For this review, take the finished solid that the model builds, in its own axes (mm). Coordinates: 2 decimals unless noted, no trailing zeros. Loops run counter-clockwise (first coordinate to the right, second up) from the corner with the lowest first, then second, coordinate; pieces in that order, holes last. Notation, with made-up numbers: (-6, 49) - (22, 49) arc R13 ccw to (22, 63) - close; hole circle Ø9 at (86.25, 42). An arc over 180 degrees is marked (long way). One line per item, written item: value. Start each with the question number.
1. Insertion check: pin 1 (1.1 mm diameter, centred on y = -11, z = 2, fed in from -X); pin 2 (4.5 mm diameter, centred on x = -129.33, y = 110, fed in from -Z); pin 3 (2 mm diameter, centred on y = 57, z = 1.5, fed in from +X). Each pin has a flat end and moves straight along its axis. Give the tip position at first contact, or say it passes through.
2. Take a section at D-D, the plane y = -95. State the section outline as (x, z) points, and give its area (3 significant figures).
3. Take a section at C-C, the plane z = 2.8. Count the separate pieces of the cut face and the enclosed holes in it, and give its area (3 significant figures).
4. Take a section at A-A, the plane y = 0. State the section outline as (x, z) points.
5. Take a section at B-B, the plane x = -3. State the section outline as (y, z) points.
6. To check wall thickness, follow line 1 (X direction, y = -18.5, z = 2.4); line 2 (Y direction, x = -54.06, z = 2.8) (3 decimals); line 3 (X direction, y = 25.5, z = 2.3). State the ranges of each line that lie inside material, in increasing order. Write a range as from..to.
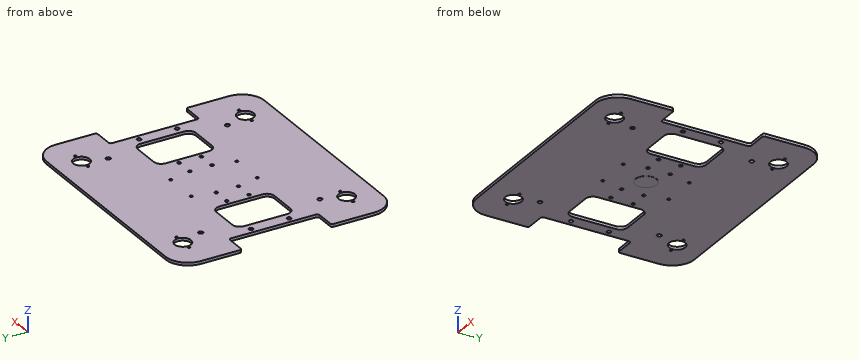
```python
from build123d import *

# Parameters (mm, degrees)
SKETCH2_R                      = 1.65
SKETCH2_R_2                    = 11
SKETCH2_R_3                    = 3
SKETCH2_R_4                    = 1.9
SKETCH2_R_5                    = 2.25
BOSS_EXTRUDE1_DEPTH            = 3.8
M5_CLEARANCE_HOLE1_D           = 5.5
M5_CLEARANCE_HOLE1_CSINK_D     = 5.55
M5_CLEARANCE_HOLE1_CSINK_ANGLE = 90
SKETCH4_R                      = 13.987722527
BOSS_EXTRUDE2_DEPTH            = 0.2


with BuildPart() as part:
    # Sketch2 → Boss-Extrude1 (new body)
    with BuildSketch(Plane.XY):
        with BuildLine():
            Line((165, 63), (165, 115))
            ThreePointArc((165, 115), (156.213203436, 136.213203436), (135, 145))
            Line((135, 145), (71.563974327, 145))
            Line((71.563974327, 145), (-71.563974327, 145))
            Line((-71.563974327, 145), (-135, 145))
            ThreePointArc((-135, 145), (-156.213203436, 136.213203436), (-165, 115))
            Line((-165, 115), (-165, 63))
            ThreePointArc((-165, 63), (-164.121320344, 60.878679656), (-162, 60))
            Line((-162, 60), (-138, 60))
            ThreePointArc((-138, 60), (-135.878679656, 59.121320344), (-135, 57))
            Line((-135, 57), (-135, -57))
            ThreePointArc((-135, -57), (-135.878679656, -59.121320344), (-138, -60))
            Line((-138, -60), (-162, -60))
            ThreePointArc((-162, -60), (-164.121320344, -60.878679656), (-165, -63))
            Line((-165, -63), (-165, -117.5))
            ThreePointArc((-165, -117.5), (-156.213203436, -138.713203436), (-135, -147.5))
            Line((-135, -147.5), (135, -147.5))
            ThreePointArc((135, -147.5), (156.213203436, -138.713203436), (165, -117.5))
            Line((165, -117.5), (165, -63))
            ThreePointArc((165, -63), (164.121320344, -60.878679656), (162, -60))
            Line((162, -60), (138, -60))
            ThreePointArc((138, -60), (135.878679656, -59.121320344), (135, -57))
            Line((135, -57), (135, 57))
            ThreePointArc((135, 57), (135.878679656, 59.121320344), (138, 60))
            Line((138, 60), (162, 60))
            ThreePointArc((162, 60), (164.121320344, 60.878679656), (165, 63))
        make_face()
        with Locations(Location((-129.334802826, -110, 0), (0, 0, 180))):
            Circle(SKETCH2_R, mode=Mode.SUBTRACT)
        with Locations(Location((-115, -110, 0), (0, 0, 180))):
            Circle(SKETCH2_R_2, mode=Mode.SUBTRACT)
        with Locations(Location((-100.665197174, -110, 0), (0, 0, 180))):
            Circle(SKETCH2_R, mode=Mode.SUBTRACT)
        with Locations(Location((-105, -80, 0), (0, 0, 180))):
            Circle(SKETCH2_R_3, mode=Mode.SUBTRACT)
        with Locations(Location((-127.121259344, -25.5, 0), (0, 0, 180))):
            Circle(SKETCH2_R, mode=Mode.SUBTRACT)
        with Locations(Location((-23.312977745, -44.325601579, 0), (0, 0, 180))):
            Circle(SKETCH2_R_4, mode=Mode.SUBTRACT)
        with Locations(Location((-54.06, -14.995, 0), (0, 0, 180))):
            Circle(SKETCH2_R_5, mode=Mode.SUBTRACT)
        with Locations(Location((-30, -14.995, 0), (0, 0, 180))):
            Circle(SKETCH2_R_5, mode=Mode.SUBTRACT)
        with Locations(Location((100.665197174, -110, 0), (0, 0, 180))):
            Circle(SKETCH2_R, mode=Mode.SUBTRACT)
        with Locations(Location((115, -110, 0), (0, 0, 180))):
            Circle(SKETCH2_R_2, mode=Mode.SUBTRACT)
        with Locations(Location((105, -80, 0), (0, 0, 180))):
            Circle(SKETCH2_R_3, mode=Mode.SUBTRACT)
        with Locations(Location((129.334802826, -110, 0), (0, 0, 180))):
            Circle(SKETCH2_R, mode=Mode.SUBTRACT)
        with Locations(Location((23.312977745, -44.325601579, 0), (0, 0, 180))):
            Circle(SKETCH2_R_4, mode=Mode.SUBTRACT)
        with Locations(Location((30, -14.995, 0), (0, 0, 180))):
            Circle(SKETCH2_R_5, mode=Mode.SUBTRACT)
        with Locations(Location((54.06, -14.995, 0), (0, 0, 180))):
            Circle(SKETCH2_R_5, mode=Mode.SUBTRACT)
        with Locations(Location((127.121259344, -25.5, 0), (0, 0, 180))):
            Circle(SKETCH2_R, mode=Mode.SUBTRACT)
        with Locations(Location((-127.121259344, 25.5, 0), (0, 0, 180))):
            Circle(SKETCH2_R, mode=Mode.SUBTRACT)
        with BuildLine():
            ThreePointArc((-117.12, 28.95), (-114.191067812, 36.021067812), (-107.12, 38.95))
            Line((-107.12, 38.95), (-71.12, 38.95))
            ThreePointArc((-71.12, 38.95), (-64.048932188, 36.021067812), (-61.12, 28.95))
            Line((-61.12, 28.95), (-61.12, -29.05))
            ThreePointArc((-61.12, -29.05), (-64.048932188, -36.121067812), (-71.12, -39.05))
            Line((-71.12, -39.05), (-107.12, -39.05))
            ThreePointArc((-107.12, -39.05), (-114.191067812, -36.121067812), (-117.12, -29.05))
            Line((-117.12, -29.05), (-117.12, 28.95))
        make_face(mode=Mode.SUBTRACT)
        with Locations(Location((-54.06, 14.895, 0), (0, 0, 180))):
            Circle(SKETCH2_R_5, mode=Mode.SUBTRACT)
        with Locations(Location((-30, 14.895, 0), (0, 0, 180))):
            Circle(SKETCH2_R_5, mode=Mode.SUBTRACT)
        with Locations(Location((-23.312977745, 44.325601579, 0), (0, 0, 180))):
            Circle(SKETCH2_R_4, mode=Mode.SUBTRACT)
        with Locations(Location((-105, 80, 0), (0, 0, 180))):
            Circle(SKETCH2_R_3, mode=Mode.SUBTRACT)
        with Locations(Location((-129.334802826, 110, 0), (0, 0, 180))):
            Circle(SKETCH2_R, mode=Mode.SUBTRACT)
        with Locations(Location((-115, 110, 0), (0, 0, 180))):
            Circle(SKETCH2_R_2, mode=Mode.SUBTRACT)
        with Locations(Location((-100.665197174, 110, 0), (0, 0, 180))):
            Circle(SKETCH2_R, mode=Mode.SUBTRACT)
        with Locations(Location((30, 14.895, 0), (0, 0, 180))):
            Circle(SKETCH2_R_5, mode=Mode.SUBTRACT)
        with Locations(Location((54.06, 14.895, 0), (0, 0, 180))):
            Circle(SKETCH2_R_5, mode=Mode.SUBTRACT)
        with Locations(Location((23.312977745, 44.325601579, 0), (0, 0, 180))):
            Circle(SKETCH2_R_4, mode=Mode.SUBTRACT)
        with BuildLine():
            Line((61.12, -29.05), (61.12, 28.95))
            ThreePointArc((61.12, 28.95), (64.048932188, 36.021067812), (71.12, 38.95))
            Line((71.12, 38.95), (107.12, 38.95))
            ThreePointArc((107.12, 38.95), (114.191067812, 36.021067812), (117.12, 28.95))
            Line((117.12, 28.95), (117.12, -29.05))
            ThreePointArc((117.12, -29.05), (114.191067812, -36.121067812), (107.12, -39.05))
            Line((107.12, -39.05), (71.12, -39.05))
            ThreePointArc((71.12, -39.05), (64.048932188, -36.121067812), (61.12, -29.05))
        make_face(mode=Mode.SUBTRACT)
        with Locations(Location((127.121259344, 25.5, 0), (0, 0, 180))):
            Circle(SKETCH2_R, mode=Mode.SUBTRACT)
        with Locations(Location((105, 80, 0), (0, 0, 180))):
            Circle(SKETCH2_R_3, mode=Mode.SUBTRACT)
        with Locations(Location((100.665197174, 110, 0), (0, 0, 180))):
            Circle(SKETCH2_R, mode=Mode.SUBTRACT)
        with Locations(Location((115, 110, 0), (0, 0, 180))):
            Circle(SKETCH2_R_2, mode=Mode.SUBTRACT)
        with Locations(Location((129.334802826, 110, 0), (0, 0, 180))):
            Circle(SKETCH2_R, mode=Mode.SUBTRACT)
    extrude(amount=BOSS_EXTRUDE1_DEPTH)

    # M5 Clearance Hole1 (through all)
    with Locations(Plane(origin=(-127.121259344, 25.5, 3.8), x_dir=(1, 0, 0), z_dir=(0, 0, 1))):
        with Locations((0, 0), (0, -51), (254.242518688, -51), (254.242518688, 0)):
            CounterSinkHole(M5_CLEARANCE_HOLE1_D / 2, M5_CLEARANCE_HOLE1_CSINK_D / 2, counter_sink_angle=M5_CLEARANCE_HOLE1_CSINK_ANGLE)

    # Sketch4 → Boss-Extrude2 (add)
    with BuildSketch(Plane(origin=(0, 0, 0), x_dir=(-1, 0, 0), z_dir=(0, 0, -1))):
        with Locations(Location((-0.021137242, 0, 0), (0, 0, 180))):
            Circle(SKETCH4_R)
    extrude(amount=BOSS_EXTRUDE2_DEPTH)


solid = part.part
```
Solutions:
1. pin 1: x = -135
1. pin 2: z = 0
1. pin 3: x = 135.17
2. outline: (-165, 0) - (165, 0) - (165, 3.8) - (-165, 3.8) - close
2. area: 1,250 mm2
3. separate pieces: 1
3. enclosed holes: 34
3. area: 78,000 mm2
4. outline: (-135, 0) - (-117.12, 0) - (-117.12, 3.8) - (-135, 3.8) - close; (-61.12, 0) - (-13.97, 0) - (-13.97, -0.2) - (14.01, -0.2) - (14.01, 0) - (61.12, 0) - (61.12, 3.8) - (-61.12, 3.8) - close; (117.12, 0) - (135, 0) - (135, 3.8) - (117.12, 3.8) - close
5. outline: (-147.5, 0) - (-13.66, 0) - (-13.66, -0.2) - (13.66, -0.2) - (13.66, 0) - (145, 0) - (145, 3.8) - (-147.5, 3.8) - close
6. line 1: -135..-117.12, -61.12..61.12, 117.12..135
6. line 2: -147.5..-17.245, -12.745..12.645, 17.145..145
6. line 3: -135..-129.87, -124.37..-117.12, -61.12..61.12, 117.12..124.37, 129.87..135
